Can you work these out from the model? Positions are in its coordinate system, mm. Coordinates: 2 decimals unless noted, no trailing zeros. Loops run counter-clockwise (first coordinate to the right, second up) from the corner with the lowest first, then second, coordinate; pieces in that order, holes last.
```python
from build123d import *

# Parameters (mm, degrees)
BOSS_EXTRUDE1_DEPTH     = 6.35
F_1_4_CLEARANCE_HOLE1_D = 6.7564
F_8_CLEARANCE_HOLE1_D   = 4.4958
FILLET1_R               = 2.54


with BuildPart() as part:
    # Sketch1 → Boss-Extrude1 (new body)
    with BuildSketch(Plane(origin=(0, 0, 0), x_dir=(1, 0, 0), z_dir=(0, 1, 0))):
        Polygon((46.634796, -31.75), (46.634796, 22.824939239), (46.634796, 37.882236802), (-40.259946838, 45.48454172), (-26.64141329, -31.75), align=None)
    extrude(amount=-BOSS_EXTRUDE1_DEPTH)

    # 1/4 Clearance Hole1 (through all)
    with Locations(Plane(origin=(0, -6.35, 0), x_dir=(-1, 0, 0), z_dir=(0, -1, 0))):
        with Locations((-21.234796, 32.832322476), (-39.1347856, -22.225), (-39.1347856, 12.482236802), (29.432583699, 37.26514381)):
            Hole(F_1_4_CLEARANCE_HOLE1_D / 2)

    # #8 Clearance Hole1 (through all)
    with Locations(Plane(origin=(0, 0, 0), x_dir=(1, 0, 0), z_dir=(0, 1, 0))):
        with Locations((12.698082155, 12.698082155), (-12.698082155, -12.698082155)):
            Hole(F_8_CLEARANCE_HOLE1_D / 2)

    # Fillet1
    fillet1_edges = [part.edges().sort_by_distance(p)[0] for p in [
        (46.634796, -3.175, 31.75),
        (-26.64141329, -3.175, 31.75),
        (-40.259946838, -3.175, -45.48454172),
        (46.634796, -3.175, -37.882236802),
    ]]
    fillet(fillet1_edges, radius=FILLET1_R)


solid = part.part
```
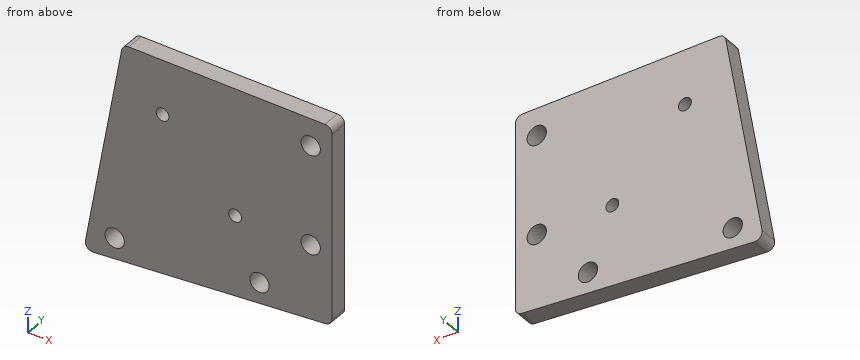
(1) I want a section at A-A on x = -12. Write out the boundary of the cut face in (y, z).
Check values:
outline: (-6.35, -43.01) - (0, -43.01) - (0, 10.56) - (-6.35, 10.56) - close; (-6.35, 14.83) - (0, 14.83) - (0, 31.75) - (-6.35, 31.75) - close
(2) I want a section at B-B on z = -31. Write out the boundary of the cut face in (x, y), then the cut area to 3 significant figures.
Check values:
outline: (-37.71, -6.35) - (18.4, -6.35) - (18.4, 0) - (-37.71, 0) - close; (24.07, -6.35) - (46.63, -6.35) - (46.63, 0) - (24.07, 0) - close
area: 500 mm2
(3) I'm going to push a flat-ended pin straight in: pin 1 (5.5 mm diameter, centred on x = -29.43, z = -37.27, fed in from +Y). Where does the tip first touch, or does it pass through?
Check values:
pin 1: passes through
(4) If I drill on probe 1 along Z at (x, y) = (39, -3); probe 2 along X at (y, z) = (-5, -10); probe 3 along Z at (x, y) = (-11, -2), over which ranges is the centre line in solid material (lowest first)?
Check values:
probe 1: z = -38.55 to -15.86, -9.11 to 18.85, 25.6 to 31.75
probe 2: x = -34 to 36.84, 41.43 to 46.63
probe 3: z = -42.92 to 11.23, 14.17 to 31.75
(5) I want a section at D-D on x = 0.5. Write out the boundary of the cut face in (y, z), then the cut area to 3 significant figures.
Check values:
outline: (-6.35, -41.92) - (0, -41.92) - (0, 31.75) - (-6.35, 31.75) - close
area: 468 mm2
(6) I want a section at C-C on y = -3. Write out the boundary of the cut face in (x, z) (3 decimals), then the cut area to 3 significant figures.
Check values:
outline: (-39.685, -42.225) arc R2.54 ccw to (-36.962, -45.196) - (44.316, -38.085) arc R2.54 ccw to (46.635, -35.555) - (46.635, 29.21) arc R2.54 ccw to (44.095, 31.75) - (-24.51, 31.75) arc R2.54 ccw to (-27.012, 29.651) - close; hole circle Ø6.756 at (-29.433, -37.265); hole circle Ø4.496 at (-12.698, 12.698); hole circle Ø4.496 at (12.698, -12.698); hole circle Ø6.756 at (21.235, -32.832); hole circle Ø6.756 at (39.135, -12.482); hole circle Ø6.756 at (39.135, 22.225)
area: 5,670 mm2
